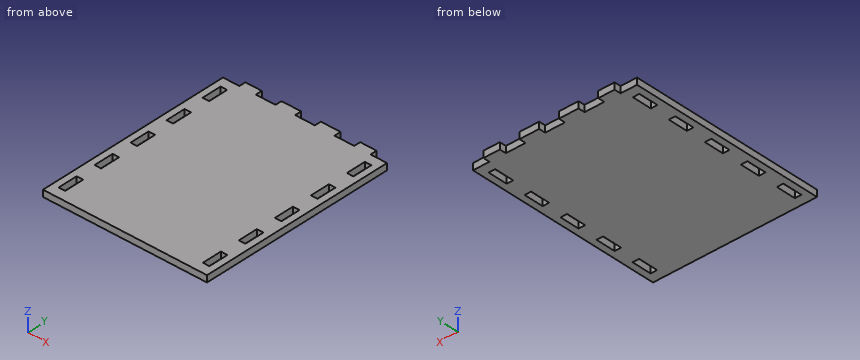
```python
from build123d import *

# Parameters (mm, degrees)
ESQUISSE1_W             = 125
ESQUISSE1_H             = 155
BOSS_EXTRU_2_DEPTH      = 5
ESQUISSE3_W             = 5
ESQUISSE3_H             = 15
ENL_V_MAT_EXTRU_1_DEPTH = 5
ESQUISSE4_W             = 15
ESQUISSE4_H             = 5
ESQUISSE4_W_2           = 12.5
ENL_V_MAT_EXTRU_2_DEPTH = 50


with BuildPart() as part:
    # Esquisse1 → Boss.-Extru.2 (new body)
    with BuildSketch(Plane.XY):
        with Locations((8.848314607, 6.994382022)):
            Rectangle(ESQUISSE1_W, ESQUISSE1_H)
    extrude(amount=BOSS_EXTRU_2_DEPTH)

    # Esquisse3 → Enlèv. mat.-Extru.1 (cut)
    with BuildSketch(Plane(origin=(0, 0, 0), x_dir=(-1, 0, 0), z_dir=(0, 0, -1))):
        with Locations((-63.848314607, -55.505617978)):
            Rectangle(ESQUISSE3_W, ESQUISSE3_H)
        with Locations((-63.848314607, -25.505617978)):
            Rectangle(ESQUISSE3_W, ESQUISSE3_H)
        with Locations((-63.848314607, 4.494382022)):
            Rectangle(ESQUISSE3_W, ESQUISSE3_H)
        with Locations((-63.848314607, 34.494382022)):
            Rectangle(ESQUISSE3_W, ESQUISSE3_H)
        with Locations((-63.848314607, 64.494382022)):
            Rectangle(ESQUISSE3_W, ESQUISSE3_H)
        with Locations((46.151685393, -55.505617978)):
            Rectangle(ESQUISSE3_W, ESQUISSE3_H)
        with Locations((46.151685393, 34.494382022)):
            Rectangle(ESQUISSE3_W, ESQUISSE3_H)
        with Locations((46.151685393, -25.505617978)):
            Rectangle(ESQUISSE3_W, ESQUISSE3_H)
        with Locations((46.151685393, 4.494382022)):
            Rectangle(ESQUISSE3_W, ESQUISSE3_H)
        with Locations((46.151685393, 64.494382022)):
            Rectangle(ESQUISSE3_W, ESQUISSE3_H)
    extrude(amount=-ENL_V_MAT_EXTRU_1_DEPTH, mode=Mode.SUBTRACT)

    # Esquisse4 → Enlèv. mat.-Extru.2 (cut)
    with BuildSketch(Plane(origin=(0, 0, 0), x_dir=(-1, 0, 0), z_dir=(0, 0, -1))):
        with Locations((-38.848314607, 81.994382022)):
            Rectangle(ESQUISSE4_W, ESQUISSE4_H)
        with Locations((-65.098314607, 81.994382022)):
            Rectangle(ESQUISSE4_W_2, ESQUISSE4_H)
        with Locations((-8.848314607, 81.994382022)):
            Rectangle(ESQUISSE4_W, ESQUISSE4_H)
        with Locations((21.151685393, 81.994382022)):
            Rectangle(ESQUISSE4_W, ESQUISSE4_H)
        with Locations((47.401685393, 81.994382022)):
            Rectangle(ESQUISSE4_W_2, ESQUISSE4_H)
    extrude(amount=-ENL_V_MAT_EXTRU_2_DEPTH, mode=Mode.SUBTRACT)


solid = part.part
```
Part model, mm, in its own coordinate system. Give positions to 0.01 mm unless a question says otherwise; leave off trailing zeros. Order: outer loops, then holes, each group sorted by start corner. A loop starts at its lowest first (then second) coordinate and runs counter-clockwise, first axis right, second up. Notation, with made-up numbers: M -37.5,3 L -21.5,3 A30 ccw -21.5,39 Z; hole C 46.25,71 d5. An arc over 180 degrees is marked long. Use a Markdown table: item, result. Add a question column.
(1) Saw through at A-A, the plane y = 63.5. Give the cut face in (x, z).
(2) Drop flat-ended pins along their axis: P1, Ø2.5, axis at x = -45.5, z = 2.5, coming from the +Y side; P2, Ø1.5, axis at x = -16.5, y = -4, coming from the -Z side; P3, Ø1.5, axis at y = 81.5, z = 3, coming from the -X side. Give the stop position or say it passes through.
(3) Probe line 1 along X through (y, z) = (68, 4.8); line 2 along Y through (x, z) = (-45.5, 2.75); line 3 along Y through (x, z) = (1.5, 0.7). List the from-to ranges inside material, lowest first. Write a range as [from, to].
(4) Saw through at B-B, the plane z = 2.35. Give the number of separate pieces and of enclosed holes in the cut face, and give its area (3 significant figures).
Answer key:
| question | item | result |
|---|---|---|
| 1 | outline | M -53.65,0 L -48.65,0 L -48.65,5 L -53.65,5 Z; M -43.65,0 L 61.35,0 L 61.35,5 L -43.65,5 Z; M 66.35,0 L 71.35,0 L 71.35,5 L 66.35,5 Z |
| 2 | P1 | y = 79.49 |
| 2 | P2 | z = 0 |
| 2 | P3 | x = -41.15 |
| 3 | line 1 | [-53.65, -48.65], [-43.65, 61.35], [66.35, 71.35] |
| 3 | line 2 | [-70.51, -63.01], [-48.01, -33.01], [-18.01, -3.01], [11.99, 26.99], [41.99, 56.99], [71.99, 79.49] |
| 3 | line 3 | [-70.51, 79.49] |
| 4 | separate pieces | 1 |
| 4 | enclosed holes | 10 |
| 4 | area | 18,300 mm^2 |
